```python
from build123d import *

# Parameters (mm, degrees)
SKETCH1_W           = 30
SKETCH1_H           = 30
BOSS_EXTRUDE1_DEPTH = 26
SHELL1_T            = -3
SKETCH3_R           = 4
CUT_EXTRUDE1_DEPTH  = 43.438190348
BOSS_EXTRUDE4_START = -15
SKETCH4_W           = 10
SKETCH4_H           = 20
BOSS_EXTRUDE4_DEPTH = 30
CUT_EXTRUDE2_DEPTH  = 10
RIB1_REACH          = 58.93
SKETCH7_WALL_W      = 122.930630432
SKETCH7_WALL_H      = 8
CUT_EXTRUDE3_DEPTH  = 10
CUT_EXTRUDE4_DEPTH  = 10
BOSS_EXTRUDE5_REACH = 51.434
SKETCH11_W          = 8
SKETCH11_H          = 10


with BuildPart() as part:
    # Sketch1 → Boss-Extrude1 (new body)
    with BuildSketch(Plane(origin=(0, 0, 0), x_dir=(1, 0, 0), z_dir=(0, 1, 0))):
        Rectangle(SKETCH1_W, SKETCH1_H)
    extrude(amount=BOSS_EXTRUDE1_DEPTH)

    # Shell1
    shell1_openings = [part.faces().sort_by_distance(p)[0] for p in [
        (-15, 13, 0),
        (15, 13, 0),
    ]]
    offset(amount=SHELL1_T, openings=shell1_openings, kind=Kind.INTERSECTION)

    # Sketch3 → Cut-Extrude1 (cut, through all)
    with BuildSketch(Plane.XY.offset(15)):
        with Locations((0, 13)):
            Circle(SKETCH3_R)
    extrude(amount=-CUT_EXTRUDE1_DEPTH, mode=Mode.SUBTRACT)

    # Sketch4 → Boss-Extrude4 (add)
    with BuildSketch(Plane(origin=(0, 0, 0), x_dir=(0, 0, -1), z_dir=(1, 0, 0)).offset(BOSS_EXTRUDE4_START)):
        with Locations((0, 36)):
            Rectangle(SKETCH4_W, SKETCH4_H)
    extrude(amount=BOSS_EXTRUDE4_DEPTH)

    # Sketch6 → Cut-Extrude2 (cut)
    with BuildSketch(Plane(origin=(0, 0, -5), x_dir=(-1, 0, 0), z_dir=(0, 0, -1))):
        with BuildLine():
            Line((15, 26), (15, 36.352761804))
            Line((15, 36.352761804), (-3.705905484, 41.364994072))
            ThreePointArc((-3.705905484, 41.364994072), (-9.829629226, 37.829459621), (-6.294095226, 31.705735619))
            Line((-6.294095226, 31.705735619), (15, 26))
        make_face()
    extrude(amount=-CUT_EXTRUDE2_DEPTH, mode=Mode.SUBTRACT)

    # Sketch7 wall → Rib1 (add, up to next)
    with BuildSketch(Plane(origin=(15, 28.5, -7.5), x_dir=(0, -0.707106781187, -0.707106781187), z_dir=(0, 0.707106781187, -0.707106781187)), mode=Mode.PRIVATE) as rib1_sk1:
        with Locations((0, 4)):
            Rectangle(SKETCH7_WALL_W, SKETCH7_WALL_H)
    rib1_tool1 = extrude(rib1_sk1.sketch, amount=-RIB1_REACH, mode=Mode.PRIVATE) - part.part
    rib1 = rib1_tool1.solids().sort_by_distance((15, 28.5, -7.5))[0]
    add(rib1)

    # Mirror1: Rib1 across plane
    add(rib1.mirror(Plane.XY))

    # Sketch8 → Cut-Extrude3 (cut)
    with BuildSketch(Plane(origin=(0, 0, -5), x_dir=(-1, 0, 0), z_dir=(0, 0, -1))):
        Polygon((15, 41.529142706), (-1.685466574, 46), (15, 46), align=None)
    extrude(amount=-CUT_EXTRUDE3_DEPTH, mode=Mode.SUBTRACT)

    # Sketch9 → Cut-Extrude4 (cut)
    with BuildSketch(Plane(origin=(0, 0, -5), x_dir=(-1, 0, 0), z_dir=(0, 0, -1))):
        with BuildLine():
            Line((-15, 36.535364751), (-15, 46))
            Line((-15, 46), (-8.228107743, 46))
            ThreePointArc((-8.228107743, 46), (-13.132683365, 42.354253071), (-15, 36.535364751))
        make_face()
    extrude(amount=-CUT_EXTRUDE4_DEPTH, mode=Mode.SUBTRACT)

    # Boss-Extrude5: up to this plane
    boss_extrude5_end = Plane(origin=(0, 34, 0), z_dir=(0, 1, 0))
    # Sketch11 → Boss-Extrude5 (add, up to the surface)
    with BuildSketch(Plane(origin=(-10.092999923, 37.667588512, 0), x_dir=(0.965925826289068, 0.25881904510252185, 0), z_dir=(0.25881904510252185, -0.965925826289068, 0)), mode=Mode.PRIVATE) as boss_extrude5_sk1:
        with Locations((-1.080100297, 0)):
            Rectangle(SKETCH11_W, SKETCH11_H)
    boss_extrude5_tool1 = split(extrude(boss_extrude5_sk1.sketch, amount=BOSS_EXTRUDE5_REACH, dir=(0, -1, 0), mode=Mode.PRIVATE), bisect_by=boss_extrude5_end, keep=Keep.BOTH, mode=Mode.PRIVATE)
    add(boss_extrude5_tool1.solids().sort_by_distance((-11.136297, 37.388038, 0))[0])


solid = part.part
```
Source: CAD feature listing. Evaluate the final solid. Frame: model axes, mm. A direction names the side the tool comes from. Round coordinates to 2 decimals unless told otherwise and drop trailing zeros. Order: outer loops, then holes, each group sorted by start corner. A loop starts at its lowest first (then second) coordinate and runs counter-clockwise, first axis right, second up. Notation, with made-up numbers: (-30, 31.5) -> (-18, 31.5) arc R6 cw to (-18, 36.5) -> close; hole circle Ø8 at (22, 70). An arc over 180 degrees is marked (long way). One line per item, written item: value. Start each with the question number.
Q1. Pin query (flat end, axial travel): pin 1 (6.5 mm diameter, centred on x = 0, y = 13, fed in from -Z); pin 2 (4 mm diameter, centred on y = 28.5, z = 7.5, fed in from -X); pin 3 (6 mm diameter, centred on x = -7.5, y = 34, fed in from -Z); pin 4 (5 mm diameter, centred on x = -5.5, z = -9.5, fed in from +Y). Return the tip coordinate at first contact, or that it passes through.
Q2. Material intervals for probe 1 along Z at (x, y) = (-1, 7.5); probe 2 along Y at (x, z) = (0, -13.95); probe 3 along Y at (x, z) = (6, -7.25), sorted ascending.
Q3. Section query B-B (z = -6.5). Return the cut outline in (x, y), plus the area to 3 significant figures.
Q4. Section query A-A (y = 13). Return the cut outline in (x, z), plus the area to 3 significant figures.
Q5. Section query D-D (x = -1). Return the cut outline in (y, z), plus the area to 3 significant figures.
Q6. Access query for faces 4 (the flat face through (7, 28, -7)), 5 (the cylindrical face through (13.1, 42.4, -0.1)), 6 (the flat face through (7, 28, 7)), 7 (the flat face through (-4, 15, 12)), 8 (the flat face through (-1.86, 39.874, -0.07)). Directions: +Z, -Z, +X, -X, +Y, -Y. A direction counts if a zero-diameter tool reaches every point of the face in a straight line with its end or side. Return the directions, or none.
Q7. Draft query along X for faces 1 (the cylindrical face through (-0.521, 16.966, 13.521)), 2 (the flat face through (0, 0, 0)), 3 (the flat face through (-4.204, 28.893, -0.07)). Return one class per face: pulls with the +X half, pulls with the -X half, needs draft (parallel to the pull), parting line crosses it, or undercut.
Q8. Section query C-C (x = -12). Return the cut outline in (y, z), plus the area to 3 significant figures.
Findings below:
1. pin 1: through
1. pin 2: x = 7
1. pin 3: z = -5
1. pin 4: y = 26
2. probe 1: -15 to -12, 12 to 15
2. probe 2: 0 to 9, 17 to 26
2. probe 3: 0 to 3, 23 to 26
3. outline: (-15, 0) -> (15, 0) -> (15, 3) -> (-15, 3) -> close; (-15, 23) -> (15, 23) -> (15, 29.5) -> (7, 29.5) -> (7, 26) -> (-15, 26) -> close
3. area: 208 mm²
4. outline: (-15, -15) -> (-4, -15) -> (-4, -12) -> (-15, -12) -> close; (-15, 12) -> (-4, 12) -> (-4, 15) -> (-15, 15) -> close; (4, -15) -> (15, -15) -> (15, -12) -> (4, -12) -> close; (4, 12) -> (15, 12) -> (15, 15) -> (4, 15) -> close
4. area: 132 mm²
5. outline: (0, -15) -> (9.13, -15) -> (9.13, -12) -> (3, -12) -> (3, 12) -> (9.13, 12) -> (9.13, 15) -> (0, 15) -> close; (16.87, -15) -> (26, -15) -> (26, -5) -> (29.75, -5) -> (29.75, 5) -> (26, 5) -> (26, 15) -> (16.87, 15) -> (16.87, 12) -> (23, 12) -> (23, -12) -> (16.87, -12) -> close; (40.1, -5) -> (45.28, -5) -> (45.28, 5) -> (40.1, 5) -> close
5. area: 343 mm²
6. face 4: -Z, -X, +Y
6. face 5: +Z, -Z, +X, +Y
6. face 6: +Z, -X, +Y
6. face 7: +X, -X
6. face 8: +Z, -Z
7. face 1: undercut
7. face 2: needs draft
7. face 3: pulls with the -X half
8. outline: (0, -15) -> (26, -15) -> (26, -5) -> (26.8, -5) -> (26.8, 5) -> (26, 5) -> (26, 15) -> (0, 15) -> close; (34, -5) -> (42.33, -5) -> (42.33, 5) -> (34, 5) -> close; hole (3, -12) -> (23, -12) -> (23, 12) -> (3, 12) -> close
8. area: 391 mm²
